Source: three-view drawing plus pictorial views. Frame: mm from the lowest corner of the part. Round coordinates to 2 decimals unless told otherwise and drop trailing zeros. Write each loop counter-clockwise with the first axis right and the second up, starting at its lowest first coordinate (ties: lowest second). Pieces come first, ordered by that corner, then holes. Notation, with made-up numbers: M 49.25,-6.75 L 59.25,-6.75 A17 ccw 59.25,7.25 Z; hole C 29,43.5 d5. An arc over 180 degrees is marked long. Answer as CSV lines item,"result". Start each with the question number.
Q1. Mould query, pull axis Y, two halves, no side actions, for the marked faces 1, 2 and 3. Classes: pulls with the +Y half, pulls with the -Y half, needs draft (parallel to the pull), parting line crosses it, or undercut.
Q2. Section query A-A on x = 165.1. Output: boundary loops of the cut face in (y, z).
Q3. First-contact query: pin 1 (1.3 mm diameter, centred on y = 15, z = 4, fed in from -X); pin 2 (5.5 mm diameter, centred on y = 10.5, z = 8, fed in from -X); pin 3 (7.5 mm diameter, centred on x = 121.5, y = 13.5, fed in from +Z). Flat tips, straight axial feed; report the tip coordinate or a pass-through.
Q4. Section query B-B on x = 19.5. Output: boundary loops of the cut face in (y, z), and give its area (3 significant figures).
Q5. Section query D-D on z = 7.5. Output: boundary loops of the cut face in (x, y), and give its area (3 significant figures).
Q6. Section query C-C on y = 23. Output: boundary loops of the cut face in (x, z), and give its area (3 significant figures).
Q7. Ray query, probe 1 along Y at (x, z) = (24.5, 7.5); probe 2 along Y at (x, z) = (31.75, 3.1); probe 3 along X at (y, z) = (5, 6.25). Return the intervals inside material, ascending.
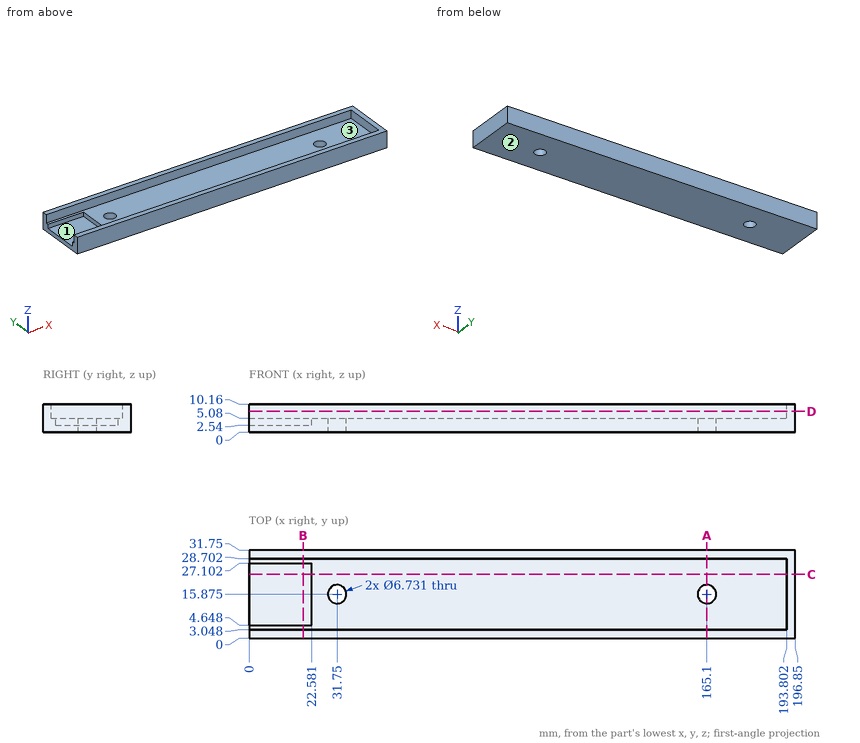
Entries:
1,face 1,"undercut"
1,face 2,"needs draft"
1,face 3,"undercut"
2,outline,"M 0,0 L 12.51,0 L 12.51,5.08 L 3.05,5.08 L 3.05,10.16 L 0,10.16 Z; M 19.24,0 L 31.75,0 L 31.75,10.16 L 28.7,10.16 L 28.7,5.08 L 19.24,5.08 Z"
3,pin 1,"stops at x = 22.58"
3,pin 2,"stops at x = 193.8"
3,pin 3,"stops at z = 5.08"
4,outline,"M 0,0 L 31.75,0 L 31.75,10.16 L 28.7,10.16 L 28.7,5.08 L 27.1,5.08 L 27.1,2.54 L 4.65,2.54 L 4.65,5.08 L 3.05,5.08 L 3.05,10.16 L 0,10.16 Z"
4,area,"135 mm^2"
5,outline,"M 0,0 L 196.85,0 L 196.85,31.75 L 0,31.75 L 0,28.7 L 193.8,28.7 L 193.8,3.05 L 0,3.05 Z"
5,area,"1,280 mm^2"
6,outline,"M 0,0 L 196.85,0 L 196.85,10.16 L 193.8,10.16 L 193.8,5.08 L 22.58,5.08 L 22.58,2.54 L 0,2.54 Z"
6,area,"958 mm^2"
7,probe 1,"y = 0 to 3.05, 28.7 to 31.75"
7,probe 2,"y = 0 to 12.51, 19.24 to 31.75"
7,probe 3,"x = 193.8 to 196.85"
